Check sheet for the modelled part. Datum: model origin and axes. Units: mm. A direction names the side the tool comes from. Coordinates: 2 decimals unless noted, no trailing zeros. Write each loop counter-clockwise with the first axis right and the second up, starting at its lowest first coordinate (ties: lowest second). Pieces come first, ordered by that corner, then holes. Notation, with made-up numbers: (13.25, 7.25) - (28.25, 7.25) arc R29 ccw to (28.25, 29.25) - close; hole circle Ø5 at (-1.5, 16). An arc over 180 degrees is marked (long way). Use one line per item in the form item = value. Start each with the question number.
1. Scan lines: line 1 along Y through (x, z) = (3.25, 0.25); line 2 along Y through (x, z) = (2.75, 0.15); line 3 along X through (y, z) = (3.5, 0.55). Record each from-to range of solid material in increasing order.
2. Draft check along X on faces 1 (the face through (0, 6.3, 1)), 2 (the face through (1.986, -7.413, 0.493)), 3 (the face through (-3.98, -4.7, 0.49)). Enter one of: +X half, -X half, draft (parallel to the pull), parting line (faces both ways), or undercut.
3. Cross-section at C-C on z = 0.2. Record the boundary of the cut face in (x, y).
4. Tool access check on faces 4 (the face through (-1.986, -7.413, 0.493)), 5 (the face through (-1.855, -6.006, 0.493)), 6 (the face through (0, 6.3, 0)). Record the directions out of +Z, -Z, +X, -X, +Y, -Y that give a thin tool (end or side, any length) a straight path to the whole face; none if there is none.
5. Cross-section at B-B on y = 3.5. Record the boundary of the cut face in (x, z), then the cut area to 3 significant figures.
6. Go/stop test with a flat-tipped pin: pin 1 Ø2 at (x, y) = (4, -2) entering from +Z. Record where the tip stops, or that it passes through.
7. Cross-section at A-A on x = -5.5. Record the boundary of the cut face in (y, z), then the cut area to 3 significant figures.
8. Cross-section at D-D on y = 6.75. Record the boundary of the cut face in (x, z), then the cut area to 4 significant figures.
```python
from build123d import *

# Parameters (mm, degrees)
BASE_EXTRUSION_DEPTH    = 1
ESQUISSE2_R             = 0.75
ENL_V_MAT_EXTRU_1_DEPTH = 2


with BuildPart() as part:
    # Esquisse1 → Base-Extrusion (new body)
    with BuildSketch(Plane.XY):
        with BuildLine():
            Line((-2.174079979, -8.113776941), (-1.793150944, -6.69213043))
            ThreePointArc((-1.793150944, -6.69213043), (-1.859468641, -5.996613305), (-2.364922946, -5.514266901))
            ThreePointArc((-2.364922946, -5.514266901), (-2.819293841, -5.296374443), (-3.253778531, -5.041123414))
            ThreePointArc((-3.253778531, -5.041123414), (-3.994900026, -4.695430516), (-4.80184043, -4.562720925))
            ThreePointArc((-4.80184043, -4.562720925), (-5.942925253, -4.168164446), (-6.649004393, -3.188776046))
            ThreePointArc((-6.649004393, -3.188776046), (-5.671041894, 3.103569646), (0, 6))
            Line((0, 6), (0, 8.4))
            ThreePointArc((0, 8.4), (-8.328136836, 1.096420015), (-2.174079979, -8.113776941))
        make_face()
    base_extrusion = extrude(amount=BASE_EXTRUSION_DEPTH)

    # Symétrie1: Base-Extrusion across Right Plane
    add(base_extrusion.mirror(Plane(origin=(0, 0, 0), x_dir=(0, 0, -1), z_dir=(1, 0, 0))))

    # Esquisse2 → Enlèv. mat.-Extru.1 (cut, through all)
    with BuildSketch(Plane.XY.offset(1)):
        with Locations((-3.25, -6.629165125)):
            Circle(ESQUISSE2_R)
    enl_v_mat_extru_1 = extrude(amount=-ENL_V_MAT_EXTRU_1_DEPTH, mode=Mode.SUBTRACT)

    # Symétrie2: Enlèv. mat.-Extru.1 across plane
    add(enl_v_mat_extru_1.mirror(Plane(origin=(0, 0, 0), x_dir=(0, 0, 1), z_dir=(1, 0, 0))), mode=Mode.SUBTRACT)


solid = part.part
```
Final values:
q1.line_1 = -7.75 to -7.38, -5.88 to -5.04, 5.2 to 7.75
q1.line_2 = -7.94 to -7.19, -6.07 to -5.33, 5.44 to 7.94
q1.line_3 = -7.64 to -5.36, 5.36 to 7.64
q2.face_1 = draft
q2.face_2 = undercut
q2.face_3 = undercut
q3.outline = (-6.65, -3.19) arc R7 cw (long way) to (6.65, -3.19) arc R2 cw to (4.8, -4.56) arc R3 ccw to (3.25, -5.04) arc R6 cw to (2.36, -5.51) arc R1 ccw to (1.79, -6.69) - (2.17, -8.11) arc R8.4 ccw (long way) to (-2.17, -8.11) - (-1.79, -6.69) arc R1 ccw to (-2.36, -5.51) arc R6 cw to (-3.25, -5.04) arc R3 ccw to (-4.8, -4.56) arc R2 cw to start; hole circle Ø1.5 at (-3.25, -6.63); hole circle Ø1.5 at (3.25, -6.63)
q4.face_4 = +Z, -Z, -Y
q4.face_5 = +Z, -Z
q4.face_6 = -Z, +X, -X, +Y, -Y
q5.outline = (-7.64, 0) - (-5.36, 0) - (-5.36, 1) - (-7.64, 1) - close; (5.36, 0) - (7.64, 0) - (7.64, 1) - (5.36, 1) - close
q5.area = 4.55 mm²
q6.pin_1 = through
q7.outline = (-6.35, 0) - (-4.42, 0) - (-4.42, 1) - (-6.35, 1) - close; (3.33, 0) - (6.35, 0) - (6.35, 1) - (3.33, 1) - close
q7.area = 4.95 mm²
q8.outline = (-5, 0) - (5, 0) - (5, 1) - (-5, 1) - close
q8.area = 10.00 mm²
